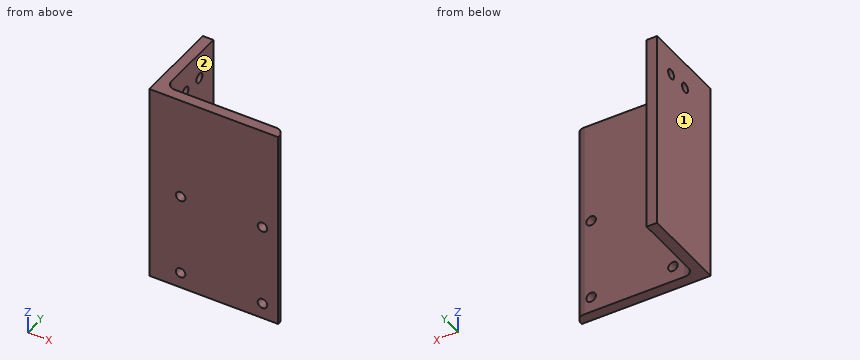
Autodesk Inventor part; units mm, degrees
ref_plane "Work Plane1" through (-74, 0, 0) normal (0.7071, -0.7071, 0) x (0, 0, 1)
ref_plane "YZ Plane" through (0, 0, 0) normal (1, 0, 0) x (0, 1, 0)
ref_plane "XZ Plane" through (0, 0, 0) normal (0, 1, 0) x (-1, 0, 0)
sketch "Sketch1" plane through (0, 0, 0) normal (0, 1, 0) x (-1, 0, 0)
  line L0 (0, 0) -> (74, 0)
  line L1 (74, 0) -> (74, -30)
  line L2 (74, -30) -> (0, -30)
  line L3 (0, -30) -> (0, 0)
  dimension "d0" = 74
  dimension "d1" = 30
extrude "Extrusion1" add sketch "Sketch1" along normal blind 6
fillet "Fillet1" radius 5 1 edges at (-74, 0, -15)
fillet "Fillet2" radius 5 1 edges at (0, 6, -15)
ref_plane "Work Plane1" through (-74, 0, 0) normal (0.7071, -0.7071, 0) x (0, 0, 1)
mirror "Mirror1" about plane through (-74, 0, 0) normal (0.7071, -0.7071, 0) of "Extrusion1", "Fillet2"
fillet "Fillet3" radius 5 1 edges at (-68, 6, -15)
sketch "Sketch5" plane through (0, 0, -30) normal (0, 0, -1) x (-1, 0, 0)
  line L0 (5, 6) -> (63, 6)
  arc A0 (5, 6) -> (0, 1) centre (5, 1) ccw
  line L1 (0, 0) -> (0, 1)
  line L2 (74, 0) -> (0, 0)
  line L3 (74, 0) -> (74, 74)
  line L4 (74, 74) -> (73, 74)
  arc A1 (73, 74) -> (68, 69) centre (73, 69) ccw
  line L5 (68, 69) -> (68, 11)
  arc A2 (63, 6) -> (68, 11) centre (63, 11) ccw
  point P0 (0, 0)
extrude "Extrusion6" add sketch "Sketch5" along normal blind 85
sketch "Sketch7" plane through (-68, 11, 0) normal (1, 0, 0) x (0, 0, -1)
  line L0 (115, 58) -> (115, 0)
  line L1 (115, 58) -> (115, 63)
  line L2 (115, -11) -> (115, 63)
  line L3 (0, 63) -> (115, 63)
  line L4 (0, 63) -> (115, 63)
  line L5 (115, 63) -> (115, 39)
  line L6 (115, 39) -> (0, 39)
  line L7 (0, 39) -> (0, 63)
  point P0 (0, -11)
  dimension "d49" = 74
  dimension "d50" = 24
extrude "Extrusion7" cut sketch "Sketch7" against normal blind 10
sketch "Sketch8" plane through (-68, 11, 0) normal (1, 0, 0) x (0, 0, -1)
  circle A0 centre (15, 13) radius 2.75
  line L0 (0, 0) -> (0, 39)
  line L1 (115, 0) -> (0, 0)
  circle A1 centre (15, 26) radius 2.75
  point P0 (0, -11)
  dimension "d53" = 5.5
  dimension "d54" = 15
  dimension "d55" = 39
  dimension "d56" = 13
  dimension "d57" = 5.5
  dimension "d58" = 15
  dimension "d59" = 26
extrude "Extrusion8" cut sketch "Sketch8" against normal blind 10
sketch "Sketch9" plane through (0, 0, 0) normal (0, -1, 0) x (1, 0, 0)
  line L0 (0, -115) -> (0, 0)
  line L1 (0, 0) -> (-74, 0)
  line L2 (-74, 0) -> (-74, -115)
  line L3 (0, -115) -> (-74, -115)
  circle A0 centre (-9, -106) radius 2.75
  circle A1 centre (-56, -106) radius 2.75
  circle A2 centre (-9, -59) radius 2.75
  circle A3 centre (-56, -59) radius 2.75
  dimension "d62" = 5.5
  dimension "d65" = 47
  dimension "d68" = 47
  dimension "d71" = 9
  dimension "d72" = 9
extrude "Extrusion9" cut sketch "Sketch9" against normal blind 10 contours A0 | A1 | A2 | A3
equation "\"d56\" = 0.333333 * d55"
equation "\"d58\" = d54"
equation "\"d59\" = 2 * d56"
equation "\"d72\" = d71"
properties part number "L_Fixer" material "Steel, Carbon"
Check sheet for the modelled part. Datum: model origin and axes. Units: mm. Face numbers are marked on the shaded views. A direction names the side the tool comes from. Give positions to 0.01 mm unless a question says otherwise; leave off trailing zeros. Write each loop counter-clockwise with the first axis right and the second up, starting at its lowest first coordinate (ties: lowest second). Pieces come first, ordered by that corner, then holes. Notation, with made-up numbers: (37.25, -30.5) - (65.25, -30.5) arc R20 ccw to (65.25, -24.5) - close; hole circle Ø1 at (30.25, -22.75). An arc over 180 degrees is marked (long way). Answer as a JSON object with one key per item and string values. Group by question number.
1) Depth check by flat-ended pin: P1, Ø9, axis at x = -9, z = -59, coming from the +Y side; P2, Ø12, axis at y = 7.5, z = -92.5, coming from the +X side; P3, Ø3, axis at x = -65, z = -66.5, coming from the +Y side. Enter the tip coordinate at first touch or a pass-through.
2) Sectioned sample at A-A (x = -56). Record the cut outline in (y, z), then the cut area to 3 significant figures.
3) Sectioned sample at D-D (z = -38). Record the cut outline in (x, y), then the cut area to 3 significant figures.
4) Sectioned sample at C-C (z = -59). Record the cut outline in (x, y).
5) Access from +Z, -Z, +X, -X, +Y, -Y to the whole of each face (thin tool, end or side, straight path). Record for the marked faces 1 and 2.
6) Sectioned sample at B-B (y = 24). Record the cut outline in (x, z).
7) Thickness scan on probe 1 along Z at (x, y) = (-56, 2); probe 2 along Y at (x, z) = (-72.25, -15); probe 3 along Y at (x, z) = (-47, -48). Record the ranges inside material, lowest first. Write a range as from..to.
Geometry results:
{
 "1": {"P1": "stops at y = 6", "P2": "stops at x = -0.03", "P3": "stops at y = 7.43"},
 "2": {"outline": "(0, -115) - (6, -115) - (6, -108.75) - (0, -108.75) - close; (0, -103.25) - (6, -103.25) - (6, -61.75) - (0, -61.75) - close; (0, -56.25) - (6, -56.25) - (6, 0) - (0, 0) - close", "area": "624 mm^2"},
 "3": {"outline": "(-74, 0) - (0, 0) - (0, 1) arc R5 ccw to (-5, 6) - (-63, 6) arc R5 cw to (-68, 11) - (-68, 50) - (-74, 50) - close", "area": "708 mm^2"},
 "4": {"outline": "(-74, 0) - (-58.75, 0) - (-58.75, 6) - (-63, 6) arc R5 cw to (-68, 11) - (-68, 50) - (-74, 50) - close; (-53.25, 0) - (-11.75, 0) - (-11.75, 6) - (-53.25, 6) - close; (-6.25, 0) - (0, 0) - (0, 1) arc R5 ccw to (-5, 6) - (-6.25, 6) - close"},
 "5": {"face 1": "+Z, -Z, -X, +Y, -Y", "face 2": "+Z, -Z, +X, +Y"},
 "6": {"outline": "(-74, -115) - (-68, -115) - (-68, -17.75) - (-74, -17.75) - close; (-74, -12.25) - (-68, -12.25) - (-68, 0) - (-74, 0) - close"},
 "7": {"probe 1": "z = -115..-108.75, -103.25..-61.75, -56.25..0", "probe 2": "y = 0..21.25, 26.75..34.25, 39.75..50", "probe 3": "y = 0..6"}
}
